Could you check a few things on this model? Use its own coordinates, in mm. Face numbers are marked on the shaded views. Give positions to 0.01 mm unless a question says otherwise; leave off trailing zeros. Write each loop counter-clockwise with the first axis right and the second up, starting at its lowest first coordinate (ties: lowest second). Pieces come first, ordered by that corner, then holes. Notation, with made-up numbers: M 88.5,-9 L 122.5,-9 A25 cw 122.5,24 Z; hole C 21,14.5 d7. An arc over 180 degrees is marked long. Answer as a JSON object with one key per item and string values. Group by question number.
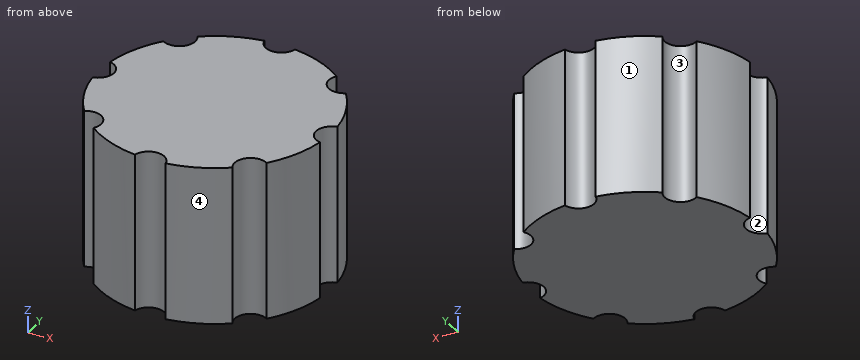
```python
from build123d import *

# Parameters (mm, degrees)
CYLINDER001_R     = 1.5
CYLINDER001_DEPTH = 20
ARRAY_COUNT       = 8
CYLINDER_R        = 11
CYLINDER_DEPTH    = 15


with BuildPart() as array:
    # Cylinder001 → Cylinder001 (new body)
    with BuildSketch(Plane(origin=(11.2, 0, 0), x_dir=(1, 0, 0), z_dir=(0, 0, 1))):
        Circle(CYLINDER001_R)
    extrude(amount=CYLINDER001_DEPTH)

    # Array: Array ×8 about axis
    array_axis = Axis((0, 0, 0), (0, 0, 1))


with BuildPart() as array_1:
    add(array.part)
    for i in range(1, ARRAY_COUNT):
        add(array.part.rotate(array_axis, i * 360 / ARRAY_COUNT))


with BuildPart() as cut:
    # Cylinder → Cylinder (new body)
    with BuildSketch(Plane.XY):
        Circle(CYLINDER_R)
    extrude(amount=CYLINDER_DEPTH)

    # Cut: cut Array
    add(array_1.part, mode=Mode.SUBTRACT)


solid = cut.part
```
1) We'd pull the mould along Y, two halves only. Please class the marked faces 1, 2, 3 and 4: released by +Y, released by -Y, zero draft, split by the parting line, or undercut.
2) If we section it at B-B, the plane x = -7: List the corners of the cut face in (y, z) for me.
3) Please list where these lines run through material, in increasing order: line 1 along X through (y, z) = (-10, 5.75); line 2 along X through (y, z) = (7.25, 13.75); line 3 along Y through (x, z) = (-5.5, 1.5). Write a range as from..to.
4) If we section it at C-C, the plane y = -6: List the corners of the cut face in (x, z) for me.
5) I'm going to push flat-ended pins straight in: pin 1 (6 mm diameter, centred on x = -2.5, z = 9.5, fed in from -Y); pin 2 (2 mm diameter, centred on y = -2.5, z = 8, fed in from +X); pin 3 (4 mm diameter, centred on y = -4, z = 4, fed in from -X); pin 4 (3 mm diameter, centred on y = 5.5, z = 12, fed in from -X). Where does each tip first touch, or does it pass through?
6) If we section it at A-A, the plane z = 10.5: List the corners of the cut face in (x, y) for me.
Taken from the geometry:
{
 "1": {"face 1": "released by +Y", "face 2": "undercut", "face 3": "undercut", "face 4": "released by -Y"},
 "2": {"outline": "M -6.73,0 L 6.73,0 L 6.73,15 L -6.73,15 Z"},
 "3": {"line 1": "-4.58..-0.9, 0.9..4.58", "line 2": "-6.58..6.58", "line 3": "-9.53..9.53"},
 "4": {"outline": "M -9.22,0 L 9.22,0 L 9.22,15 L -9.22,15 Z"},
 "5": {"pin 1": "y = -10.9", "pin 2": "x = 10.9", "pin 3": "x = -10.82", "pin 4": "x = -10.25"},
 "6": {"outline": "M -10.9,-1.47 A11 ccw -8.75,-6.67 A1.5 cw -6.67,-8.75 A11 ccw -1.47,-10.9 A1.5 cw 1.47,-10.9 A11 ccw 6.67,-8.75 A1.5 cw 8.75,-6.67 A11 ccw 10.9,-1.47 A1.5 cw 10.9,1.47 A11 ccw 8.75,6.67 A1.5 cw 6.67,8.75 A11 ccw 1.47,10.9 A1.5 cw -1.47,10.9 A11 ccw -6.67,8.75 A1.5 cw -8.75,6.67 A11 ccw -10.9,1.47 A1.5 cw Z"}
}
